Autodesk Inventor part; units mm, degrees
ref_plane "YZ Plane" through (0, 0, 0) normal (1, 0, 0) x (0, 1, 0)
ref_plane "XZ Plane" through (0, 0, 0) normal (0, 1, 0) x (-1, 0, 0)
ref_plane "XY Plane" through (0, 0, 0) normal (0, 0, 1) x (1, 0, 0)
sketch "Sketch1" plane through (0, 0, 0) normal (0, 1, 0) x (-1, 0, 0)
  circle A0 centre (0, 0) radius 2.5
  circle A1 centre (0, 0) radius 4.75
  line L0 (3, 3) -> (-3, 3)
  line L1 (-3, 3) -> (-3, -3)
  line L2 (-3, -3) -> (3, -3)
  line L3 (3, -3) -> (3, 3)
  line L4 (3, 3) -> (-3, -3) construction
  line L5 (-3, 3) -> (3, -3) construction
  line L6 (6, 6) -> (-6, 6)
  line L7 (-6, 6) -> (-6, -6)
  line L8 (-6, -6) -> (6, -6)
  line L9 (6, -6) -> (6, 6)
  line L10 (6, 6) -> (-6, -6) construction
  line L11 (-6, 6) -> (6, -6) construction
  line L12 (9, 9) -> (-9, 9)
  line L13 (-9, 9) -> (-9, -9)
  line L14 (-9, -9) -> (9, -9)
  line L15 (9, -9) -> (9, 9)
  line L16 (9, 9) -> (-9, -9) construction
  line L17 (-9, 9) -> (9, -9) construction
  dimension "d9" = 5
  dimension "d10" = 9.5
  dimension "d11" = 6
  dimension "d12" = 6
  dimension "d13" = 12
  dimension "d14" = 12
  dimension "d15" = 18
extrude "Extrusion1" add sketch "Sketch1" against normal blind 2 contours A0 | A1 | L3 L2 L1 L0 | L9 L8 L7 L6 | L15 L14 L13 L12
extrude "Extrusion2" add sketch "Sketch1" along normal blind 3.5 contours L9 L8 L7 L6
extrude "Extrusion3" add sketch "Sketch1" along normal blind 11.5 contours A1
extrude "Extrusion4" add sketch "Sketch1" along normal blind 9.5 contours L3 L2 L1 L0
extrude "Extrusion5" add sketch "Sketch1" along normal blind 4.5 contours A0
equation "\"d13\" = PIVOT_SQUARE"
equation "\"d14\" = PIVOT_SQUARE"
properties part number "HexPivot"
Work out the finished part from the listing and answer in its coordinate system (mm). A direction names the side the tool comes from. Round coordinates to 2 decimals unless told otherwise and drop trailing zeros. Loops run counter-clockwise (first coordinate to the right, second up) from the corner with the lowest first, then second, coordinate; pieces in that order, holes last. Notation, with made-up numbers: (-35, 32) - (-31, 32) arc R26 ccw to (-31, 71) - close; hole circle Ø4 at (-9, 41). An arc over 180 degrees is marked (long way). One line per item, written item: value.
Q1. Find section A-A on z = 0. Give the vertices of the cut face in (x, y), and give its area (3 significant figures).
Check values:
outline: (-9, -2) - (9, -2) - (9, 0) - (6, 0) - (6, 3.5) - (4.75, 3.5) - (4.75, 11.5) - (3, 11.5) - (3, 9.5) - (2.5, 9.5) - (2.5, 4.5) - (-2.5, 4.5) - (-2.5, 9.5) - (-3, 9.5) - (-3, 11.5) - (-4.75, 11.5) - (-4.75, 3.5) - (-6, 3.5) - (-6, 0) - (-9, 0) - close
area: 117 mm2
Q2. Find section B-B on x = 5.5. Give the vertices of the cut face in (y, z).
Check values:
outline: (-2, -9) - (0, -9) - (0, -6) - (3.5, -6) - (3.5, 6) - (0, 6) - (0, 9) - (-2, 9) - close
Q3. The mould has two halves that part along Z. Classify faces 5 (the flat face through (0, 2, 6)), 6 (the flat face through (-9, -1, 0)), 7 (the flat face through (3, 10, 0)): +Z half, -Z half, draft (parallel to the pull), parting line (faces both ways), or undercut.
Check values:
face 5: +Z half
face 6: draft
face 7: undercut
Q4. Straight lines are drawn through the part: probe 1 along Z at (x, y) = (0, 8.15); probe 2 along Y at (x, z) = (5, -7.25); probe 3 along X at (y, z) = (1.25, 1). For each, find the intervals that lie inside material, in ascending order.
Check values:
probe 1: -4.75 to -2.5, 2.5 to 4.75
probe 2: -2 to 0
probe 3: -6 to 6
Q5. Find section C-C on y = 9.75. Give the vertices of the cut face in (x, z), and give its area (3 significant figures).
Check values:
outline: circle Ø9.5 at (0, 0); hole (-3, -3) - (3, -3) - (3, 3) - (-3, 3) - close
area: 34.9 mm2
Q6. Each of these flat-tipped pins is pushed along its axis until it touches: pin 1 Ø2 at (y, z) = (11, 1) entering from -X; pin 2 Ø1.8 at (y, z) = (1, 1) entering from -X; pin 3 Ø1 at (y, z) = (9, 0.5) entering from +X. Where does it stop, or does it pass through?
Check values:
pin 1: x = -4.75
pin 2: x = -6
pin 3: x = 4.75
Q7. For faces 1 (the flat face through (0, -2, 0)), 2 (the flat face through (0, 2, -6)), 3 (the flat face through (-3, 10, 0)), 4 (the flat face through (-6, 2, 0)), determine the directions among +Z, -Z, +X, -X, +Y, -Y from which every point of the face is accessible in a straight line to the end or side of a thin tool.
Check values:
face 1: +Z, -Z, +X, -X, -Y
face 2: -Z, +X, -X, +Y
face 3: +Y
face 4: +Z, -Z, -X, +Y
Q8. Find section D-D on y = 0.5. Give the vertices of the cut face in (x, z), and give its area (3 significant figures).
Check values:
outline: (-6, -6) - (6, -6) - (6, 6) - (-6, 6) - close
area: 144 mm2
